Geometry check sheet. Reference: drawing and pictorial views, mm from the part's lowest x, y, z. A direction names the side the tool comes from. Coordinates: 2 decimals unless noted, no trailing zeros. Loops run counter-clockwise (first coordinate to the right, second up) from the corner with the lowest first, then second, coordinate; pieces in that order, holes last. Notation, with made-up numbers: (46.5, -19) - (89.5, -19) arc R30 cw to (89.5, 11) - close; hole circle Ø6 at (3.25, 30.25). An arc over 180 degrees is marked (long way). One line per item, written item: value.
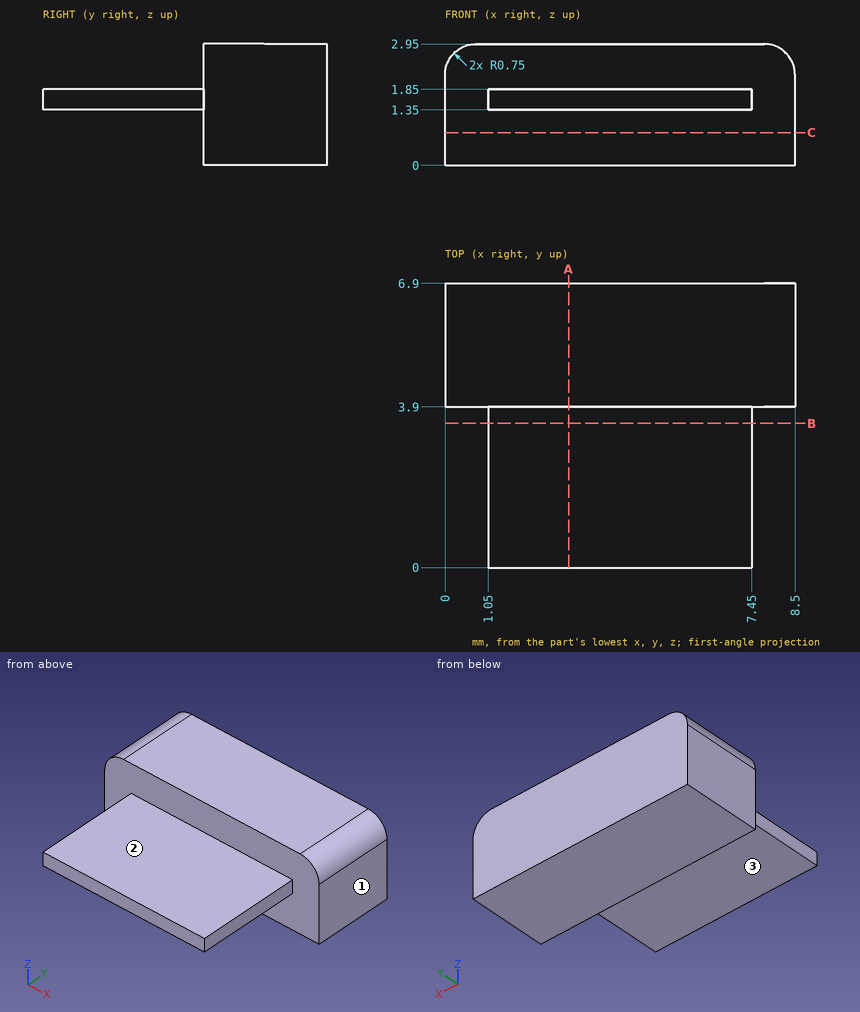
(1) Material ranges on probe 1 along Y at (x, z) = (8, 0.15); probe 2 along Z at (x, y) = (2.5, 3.75), recorded low to high. Write a range as from..to.
Reply:
probe 1: 3.9..6.9
probe 2: 1.35..1.85
(2) Access from +Z, -Z, +X, -X, +Y, -Y to the whole of each face (thin tool, end or side, straight path). Record for the marked faces 1, 2 and 3.
Reply:
face 1: +Z, -Z, +X, +Y, -Y
face 2: +Z, +X, -X, -Y
face 3: -Z, +X, -X, -Y
(3) Cross-section at A-A on x = 3. Record the cut outline in (y, z).
Reply:
outline: (0, 1.35) - (3.9, 1.35) - (3.9, 0) - (6.9, 0) - (6.9, 2.95) - (3.9, 2.95) - (3.9, 1.85) - (0, 1.85) - close
(4) Cross-section at B-B on y = 3.5. Record the cut outline in (x, z).
Reply:
outline: (1.05, 1.35) - (7.45, 1.35) - (7.45, 1.85) - (1.05, 1.85) - close
(5) Go/stop test with flat-tipped pins: pin 1 Ø3 at (x, y) = (4, 1.5) entering from -Z; pin 2 Ø0.6 at (y, z) = (1.5, 1.5) entering from -X; pin 3 Ø3 at (x, y) = (4.5, 1) entering from +Z. Record where each tip stops, or that it passes through.
Reply:
pin 1: z = 1.35
pin 2: x = 1.05
pin 3: z = 1.85
(6) Cross-section at C-C on z = 0.8. Record the cut outline in (x, y).
Reply:
outline: (0, 3.9) - (8.5, 3.9) - (8.5, 6.9) - (0, 6.9) - close
